Geometry check sheet. Reference: the model listing, model coordinates, mm. A direction names the side the tool comes from. Coordinates: 2 decimals unless noted, no trailing zeros. Loops run counter-clockwise (first coordinate to the right, second up) from the corner with the lowest first, then second, coordinate; pieces in that order, holes last. Notation, with made-up numbers: (55.5, 23.25) - (80.5, 23.25) arc R22 cw to (80.5, 29.25) - close; hole circle Ø6 at (-35, -3). An arc over 180 degrees is marked (long way). Write each question's results on one line, items separated by ' | '. Start each with the question number.
(1) Material ranges on probe 1 along X at (y, z) = (188, -2.75); probe 2 along Y at (x, z) = (2.5, -6); probe 3 along Y at (x, z) = (28, -6), recorded low to high.
(2) Go/stop test with flat-tipped pins: pin 1 Ø4 at (x, y) = (-115.75, 51.862) entering from -Z; pin 2 Ø3 at (x, y) = (7.112, 188) entering from +Z. Record where each tip stops, or that it passes through.
(3) Access from +Z, -Z, +X, -X, +Y, -Y to the whole of each face (thin tool, end or side, straight path). Record for faces 1 (the face through (-42, -20, -4)), 2 (the face through (0, -8, -4)).
(4) Sectioned sample at B-B (x = -80). Enter the section's corners in (y, z).
(5) Mould release check, pull along Y, two halves, no side actions. Record for faces 3 (the face through (114.719, -11.475, -3.506)), 4 (the face through (-2, 260, -4)), 5 (the face through (39.9, 71.9, -3.5)): pulls with the +Y half, pulls with the -Y half, needs draft (parallel to the pull), parting line crosses it, or undercut.
(6) Sectioned sample at A-A (x = -125). Enter the section's corners in (y, z).
(7) Sectioned sample at C-C (z = -5). State how many separate pieces and enclosed holes the cut face has, plus the area to 3 significant figures.
from build123d import *

# Parameters (mm, degrees)
SKETCH1_W           = 314.224
SKETCH1_H           = 280
BOSS_EXTRUDE1_DEPTH = 7.112
SKETCH2_R           = 2.5
CUT_EXTRUDE1_DEPTH  = 304.866353991
SKETCH3_R           = 2.5
CUT_EXTRUDE2_DEPTH  = 6.731
SKETCH6_R           = 8
CUT_EXTRUDE5_DEPTH  = 304.866353991
LPATTERN1_COUNT     = 4
LPATTERN1_PITCH     = 65
CUT_EXTRUDE3_DEPTH  = 304.866353991
CUT_EXTRUDE4_DEPTH  = 304.866353991
FILLET1_R           = 120
FILLET2_R           = 20
FILLET3_R           = 4


with BuildPart() as part:
    # Sketch1 → Boss-Extrude1 (new body)
    with BuildSketch(Plane(origin=(0, 0, 0), x_dir=(1, 0, 0), z_dir=(0, 0, -1))):
        with Locations((0, -120)):
            Rectangle(SKETCH1_W, SKETCH1_H)
    extrude(amount=BOSS_EXTRUDE1_DEPTH)

    # Sketch2 → Cut-Extrude1 (cut, through all)
    with BuildSketch(Plane.XY):
        with Locations((-115.75, 123.362)):
            Circle(SKETCH2_R)
        with Locations((-44.25, 123.362)):
            Circle(SKETCH2_R)
        with Locations((-35.75, 123.362)):
            Circle(SKETCH2_R)
        with Locations(Location((-115.75, 51.862, 0), (0, 0, 180))):
            Circle(SKETCH2_R)
        with Locations(Location((-44.25, 51.862, 0), (0, 0, 180))):
            Circle(SKETCH2_R)
        with Locations(Location((-35.75, 51.862, 0), (0, 0, 180))):
            Circle(SKETCH2_R)
        with Locations((115.75, 51.862)):
            Circle(SKETCH2_R)
        with Locations((44.25, 51.862)):
            Circle(SKETCH2_R)
        with Locations((35.75, 51.862)):
            Circle(SKETCH2_R)
        with Locations(Location((35.75, 123.362, 0), (0, 0, 180))):
            Circle(SKETCH2_R)
        with Locations(Location((44.25, 123.362, 0), (0, 0, 180))):
            Circle(SKETCH2_R)
        with Locations(Location((115.75, 123.362, 0), (0, 0, 180))):
            Circle(SKETCH2_R)
        with BuildLine():
            ThreePointArc((33.11827957, 107.244359979), (0, 126.112), (-33.11827957, 107.244359979))
            ThreePointArc((-33.11827957, 107.244359979), (-40, 103.323811403), (-46.88172043, 107.244359979))
            ThreePointArc((-46.88172043, 107.244359979), (-118.5, 87.612), (-46.88172043, 67.979640021))
            ThreePointArc((-46.88172043, 67.979640021), (-40, 71.900188597), (-33.11827957, 67.979640021))
            ThreePointArc((-33.11827957, 67.979640021), (0, 49.112), (33.11827957, 67.979640021))
            ThreePointArc((33.11827957, 67.979640021), (40, 71.900188597), (46.88172043, 67.979640021))
            ThreePointArc((46.88172043, 67.979640021), (118.5, 87.612), (46.88172043, 107.244359979))
            ThreePointArc((46.88172043, 107.244359979), (40, 103.323811403), (33.11827957, 107.244359979))
        make_face()
    extrude(amount=-CUT_EXTRUDE1_DEPTH, mode=Mode.SUBTRACT)

    # Sketch3 → Cut-Extrude2 (cut)
    with BuildSketch(Plane.XY):
        with Locations((137.112, 188)):
            Circle(SKETCH3_R)
        with Locations((93.225547391, 240.301837563)):
            Circle(SKETCH3_R)
    cut_extrude2 = extrude(amount=-CUT_EXTRUDE2_DEPTH, mode=Mode.SUBTRACT)

    # Sketch6 → Cut-Extrude5 (cut, through all)
    with BuildSketch(Plane(origin=(0, 0, -7.112), x_dir=(-1, 0, 0), z_dir=(0, 0, -1))):
        with Locations((-125, 27.112)):
            Circle(SKETCH6_R)
        with Locations((-95, 27.112)):
            Circle(SKETCH6_R)
        with Locations(Location((95, 27.112, 0), (0, 0, 180))):
            Circle(SKETCH6_R)
        with Locations(Location((125, 27.112, 0), (0, 0, 180))):
            Circle(SKETCH6_R)
    extrude(amount=-CUT_EXTRUDE5_DEPTH, mode=Mode.SUBTRACT)

    # LPattern1: Cut-Extrude2 ×4
    with Locations(*[(-i * LPATTERN1_PITCH, 0, 0) for i in range(1, LPATTERN1_COUNT)]):
        add(cut_extrude2, mode=Mode.SUBTRACT)

    # Sketch4 → Cut-Extrude3 (cut, through all)
    with BuildSketch(Plane.XY):
        with BuildLine():
            Line((-12, -8), (12, -8))
            ThreePointArc((12, -8), (14.121320344, -7.121320344), (15, -5))
            Line((15, -5), (15, -3))
            ThreePointArc((15, -3), (14.121320344, -0.878679656), (12, 0))
            Line((12, 0), (-12, 0))
            ThreePointArc((-12, 0), (-14.121320344, -0.878679656), (-15, -3))
            Line((-15, -3), (-15, -5))
            ThreePointArc((-15, -5), (-14.121320344, -7.121320344), (-12, -8))
        make_face()
    extrude(amount=-CUT_EXTRUDE3_DEPTH, mode=Mode.SUBTRACT)

    # Sketch5 → Cut-Extrude4 (cut, through all)
    with BuildSketch(Plane.XY):
        Polygon((66.371490886, -20), (157.112, -4), (157.112, -20), align=None)
    extrude(amount=-CUT_EXTRUDE4_DEPTH, mode=Mode.SUBTRACT)

    # Fillet1
    fillet1_edges = [part.edges().sort_by_distance(p)[0] for p in [
        (66.371490886, -20, -3.556),
    ]]
    fillet(fillet1_edges, radius=FILLET1_R)

    # Fillet2
    fillet2_edges = [part.edges().sort_by_distance(p)[0] for p in [
        (-157.112, -20, -3.556),
    ]]
    fillet(fillet2_edges, radius=FILLET2_R)

    # Fillet3
    fillet3_edges = [part.edges().sort_by_distance(p)[0] for p in [
        (157.112, -4, -3.556),
    ]]
    fillet(fillet3_edges, radius=FILLET3_R)


solid = part.part
Outcome:
1) probe 1: x = -157.11 to -60.39, -55.39 to 4.61, 9.61 to 69.61, 74.61 to 134.61, 139.61 to 157.11 | probe 2: y = -20 to -8, 0 to 49.19, 126.03 to 260 | probe 3: y = -20 to 61.19, 114.04 to 237.81, 242.79 to 260
2) pin 1: passes through | pin 2: stops at z = -6.73
3) face 1: +Z, -Z, +X, -X, -Y | face 2: +Z, -Z
4) outline: (-20, -7.11) - (49.11, -7.11) - (49.11, 0) - (-20, 0) - close; (126.11, -7.11) - (260, -7.11) - (260, 0) - (126.11, 0) - close
5) face 3: pulls with the -Y half | face 4: pulls with the +Y half | face 5: undercut
6) outline: (-20, -7.11) - (19.11, -7.11) - (19.11, 0) - (-20, 0) - close; (35.11, -7.11) - (260, -7.11) - (260, 0) - (35.11, 0) - close
7) separate pieces: 1 | enclosed holes: 26 | area: 71,400 mm2
